Could you check a few things on this drawing? It's one solid part, dimensions in mm from its lowest x, y, z. A direction names the side the tool comes from. Round coordinates to 2 decimals unless told otherwise and drop trailing zeros. Loops run counter-clockwise (first coordinate to the right, second up) from the corner with the lowest first, then second, coordinate; pieces in that order, holes last. Notation, with made-up numbers: M 69,31 L 100,31 A25 cw 100,70 Z; hole C -5.5,64 d7. An arc over 180 degrees is marked long. Use a Markdown table: item, result. Add a question column.
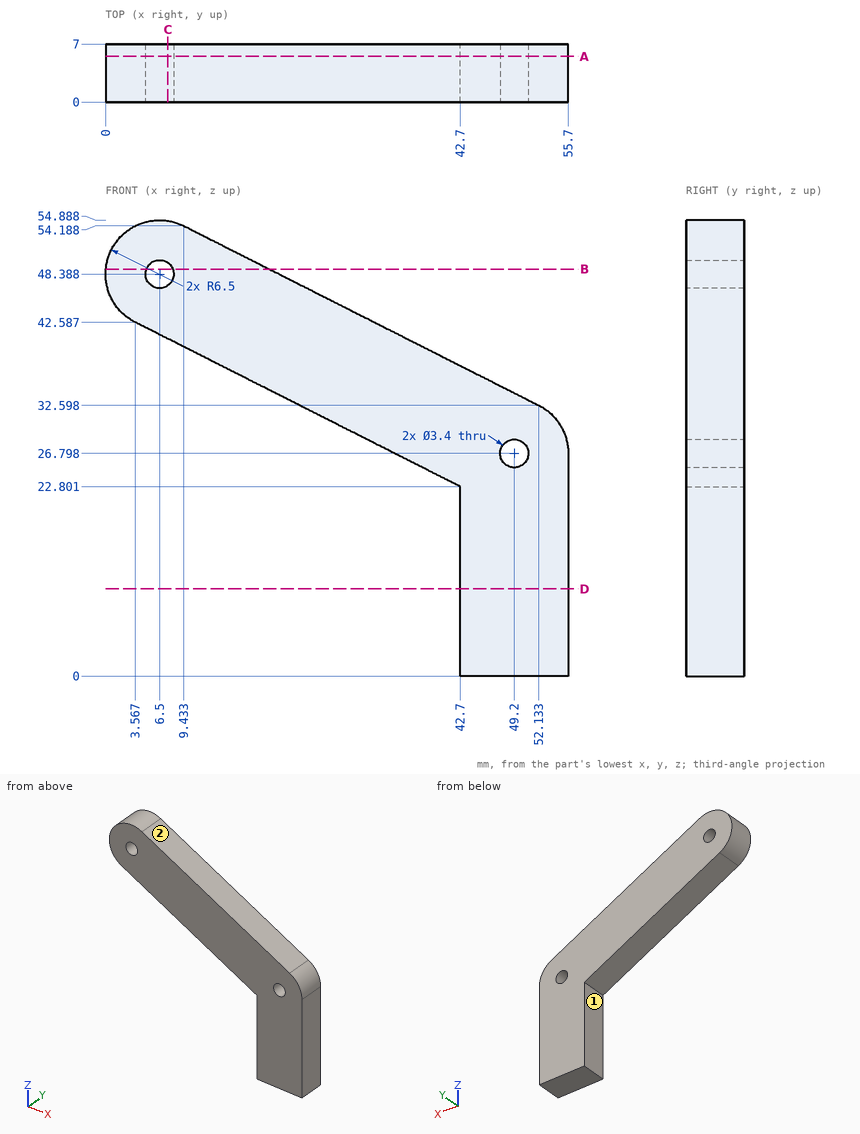
(1) Suppose I cut it at C-C on x = 7.5. List the corners of the cut face in (y, z) for me.
(2) Suppose I cut it at D-D on z = 10.5. List the corners of the cut face in (x, y) for me, and give its area (3 significant figures).
(3) Suppose I cut it at B-B on z = 49. List the corners of the cut face in (x, y) for me (1 decimal).
(4) On a 3-axis mill with a long thin cutter (end or side, diameter ignored), from which of +Z, -Z, +X, -X, +Y, -Y can I reach the whole of each face in a straight line? I mean the marked faces 1 and 2. Say none if no direction works.
(5) I'm going to push flat-ended pins straight in: pin 1 (8 mm diameter, centred on x = 28, z = 33.5, fed in from -Y); pin 2 (2 mm diameter, centred on x = 24, y = 4.5, fed in from +Z). Where does each tip first touch, or does it pass through?
(6) If I drill on probe 1 along X at (y, z) = (4.75, 11.5); probe 2 along Z at (x, y) = (49.2, 3.5); probe 3 along X at (y, z) = (5.75, 27) (1 decimal), over which ranges is the centre line in solid material (lowest first)? Write a range as [from, to].
(7) Suppose I cut it at A-A on y = 5.5. List the corners of the cut face in (x, z) for me.
Results below:
| question | item | result |
|---|---|---|
| 1 | outline | M 0,40.6 L 7,40.6 L 7,47.01 L 0,47.01 Z; M 0,49.76 L 7,49.76 L 7,54.81 L 0,54.81 Z |
| 2 | outline | M 42.7,0 L 55.7,0 L 55.7,7 L 42.7,7 Z |
| 2 | area | 91.0 mm² |
| 3 | outline | M 0,0 L 4.9,0 L 4.9,7 L 0,7 Z; M 8.1,0 L 19.7,0 L 19.7,7 L 8.1,7 Z |
| 4 | face 1 | -Z, -X, +Y, -Y |
| 4 | face 2 | +Z, +X, +Y, -Y |
| 5 | pin 1 | stops at y = 0 |
| 5 | pin 2 | stops at z = 47.33 |
| 6 | probe 1 | x = [42.7, 55.7] |
| 6 | probe 2 | z = [0, 25.1], [28.5, 34.08] |
| 6 | probe 3 | x = [34.4, 47.5], [50.9, 55.7] |
| 7 | outline | M 3.57,42.59 L 42.7,22.8 L 42.7,0 L 55.7,0 L 55.7,26.8 A6.5 ccw 52.13,32.6 L 9.43,54.19 A6.5 ccw Z; hole C 6.5,48.39 d3.4; hole C 49.2,26.8 d3.4 |
